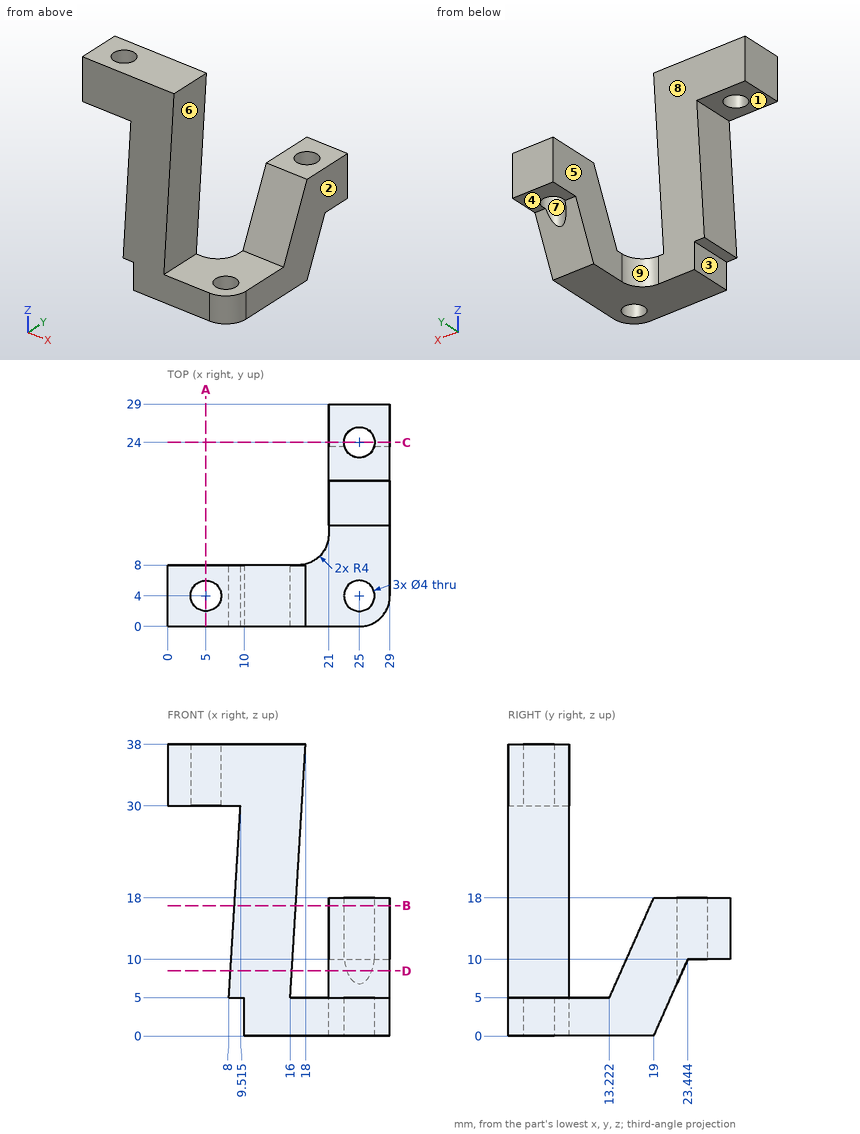
Can you work these out from the drawing? Everything is in mm from the part's minimum corner. A direction names the side the tool comes from. Coordinates: 2 decimals unless noted, no trailing zeros. Order: outer loops, then holes, each group sorted by start corner. A loop starts at its lowest first (then second) coordinate and runs counter-clockwise, first axis right, second up. Notation, with made-up numbers: M 50.5,66.25 L 87.5,66.25 A14 ccw 87.5,81.25 Z; hole C -10.5,24 d1. An arc over 180 degrees is marked long. Answer as CSV lines item,"result". Start each with the question number.
1. For pin 1 (2.5 mm diameter, centred on y = 5, z = 3, fed in from -X); pin 2 (12 mm diameter, centred on y = 7.5, z = 4.5, fed in from -X); pin 3 (6.5 mm diameter, centred on x = 26, y = 23, fed in from +Z), each with a flat end and sliding along its axis, tell me the tip position at first contact or that it passes through.
2. I want a section at A-A, the plane x = 5. Write out the boundary of the cut face in (y, z).
3. I want a section at D-D, the plane z = 8.5. Write out the boundary of the cut face in (x, y), and give its area (3 significant figures).
4. On a 3-axis mill with a long thin cutter (end or side, diameter ignored), from which of +Z, -Z, +X, -X, +Y, -Y can I reach the whole of each face in a straight line? I mean the marked faces 1, 2, 3, 4 and 5. Say none if no direction works.
5. We'd pull the mould along X, two halves only. Please class the marked faces 6, 7, 8 and 9: released by +X, released by -X, zero draft, split by the parting line, or undercut.
6. I want a section at B-B, the plane z = 17. Write out the boundary of the cut face in (x, y) (1 decimal), and give its area (3 significant figures).
7. I want a section at C-C, the plane y = 24. Write out the boundary of the cut face in (x, z), and give its area (3 significant figures).
8. I need wall thicknesses on line 1 (Y direction, x = 5, z = 35); line 2 (Z direction, x = 27.75, y = 5); line 3 (Y direction, x = 15.5, z = 25). Which ranges of each line are inside material? Lowest first, please. Write a range as [from, to].
Recorded:
1,pin 1,"stops at x = 10"
1,pin 2,"stops at x = 8"
1,pin 3,"stops at z = 18"
2,outline,"M 0,30 L 2,30 L 2,38 L 0,38 Z; M 6,30 L 8,30 L 8,38 L 6,38 Z"
3,outline,"M 8.21,0 L 16.21,0 L 16.21,8 L 8.21,8 Z; M 21,14.78 L 29,14.78 L 29,22.78 L 26.58,22.78 A2 cw 23.42,22.78 L 21,22.78 Z"
3,area,"126 mm2"
4,face 1,"-X, +Y, -Y"
4,face 2,"+Z, -Z, +X, +Y, -Y"
4,face 3,"-Z, -X, +Y, -Y"
4,face 4,"-Z, +X, -X, +Y"
4,face 5,"+Z, -Z, -X, +Y"
5,face 6,"released by +X"
5,face 7,"undercut"
5,face 8,"zero draft"
5,face 9,"released by -X"
6,outline,"M 8.7,0 L 16.7,0 L 16.7,8 L 8.7,8 Z; M 21,18.6 L 29,18.6 L 29,29 L 21,29 Z; hole C 25,24 d4"
6,area,"135 mm2"
7,outline,"M 21,10 L 23,10 L 23,18 L 21,18 Z; M 27,10 L 29,10 L 29,18 L 27,18 Z"
7,area,"32.0 mm2"
8,line 1,"y = [0, 2], [6, 8]"
8,line 2,"z = [0, 5]"
8,line 3,"y = [0, 8]"
